```python
from build123d import *

# Parameters (mm, degrees)
SKETCH1_R           = 2
BOSS_EXTRUDE1_DEPTH = 3
SKETCH2_R           = 0.75
CUT_EXTRUDE1_DEPTH  = 17.126356976


with BuildPart() as part:
    # Sketch1 → Boss-Extrude1 (new body)
    with BuildSketch(Plane(origin=(0, 0, 0), x_dir=(0, 0, -1), z_dir=(1, 0, 0))):
        with BuildLine():
            Line((-4, 10), (-4, 0))
            ThreePointArc((-4, 0), (-0.694592711, -3.939231012), (3.758770483, -1.368080573))
            Line((3.758770483, -1.368080573), (7.178971916, 8.028845635))
            ThreePointArc((7.178971916, 8.028845635), (7.045432581, 11.087399255), (4.788282007, 13.155696691))
            ThreePointArc((4.788282007, 13.155696691), (2.431074487, 13.787308542), (0, 14))
            ThreePointArc((0, 14), (-2.828427125, 12.828427125), (-4, 10))
        make_face()
        Circle(SKETCH1_R, mode=Mode.SUBTRACT)
        with Locations((0, 10)):
            Circle(SKETCH1_R, mode=Mode.SUBTRACT)
    extrude(amount=BOSS_EXTRUDE1_DEPTH)

    # Sketch2 → Cut-Extrude1 (cut, through all)
    with BuildSketch(Plane(origin=(3, 0, 0), x_dir=(0, 0, -1), z_dir=(1, 0, 0))):
        with Locations((5, 8)):
            Circle(SKETCH2_R)
    extrude(amount=-CUT_EXTRUDE1_DEPTH, mode=Mode.SUBTRACT)


solid = part.part
```
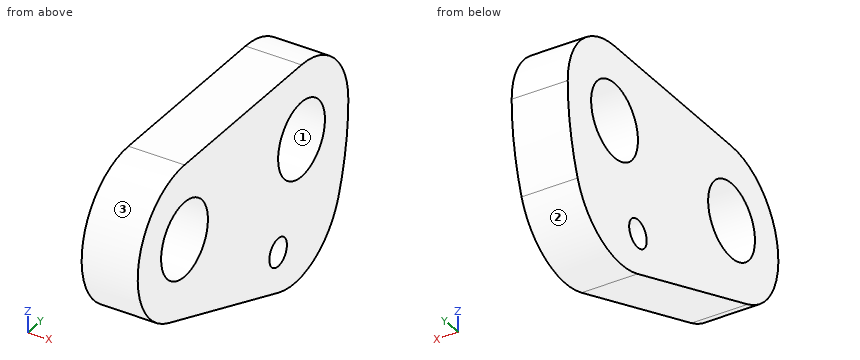
Geometry check sheet. Reference: the model listing, model coordinates, mm. Face numbers are marked on the shaded views. Coordinates: 2 decimals unless noted, no trailing zeros. Order: outer loops, then holes, each group sorted by start corner. A loop starts at its lowest first (then second) coordinate and runs counter-clockwise, first axis right, second up.
Q1. Sectioned sample at B-B on z = -1.5. Record the cut outline in (x, y).
Reply:
outline: (0, -3.71) - (3, -3.71) - (3, -1.32) - (0, -1.32) - close; (0, 1.32) - (3, 1.32) - (3, 8.68) - (0, 8.68) - close; (0, 11.32) - (3, 11.32) - (3, 13.92) - (0, 13.92) - close
Q2. Sectioned sample at D-D on z = -5. Record the cut outline in (x, y).
Reply:
outline: (0, 2.04) - (3, 2.04) - (3, 7.25) - (0, 7.25) - close; (0, 8.75) - (3, 8.75) - (3, 13.07) - (0, 13.07) - close
Q3. Sectioned sample at C-C on y = 0.5. Record the cut outline in (x, z), and give its area (3 significant figures).
Reply:
outline: (0, -4.44) - (3, -4.44) - (3, -1.94) - (0, -1.94) - close; (0, 1.94) - (3, 1.94) - (3, 4) - (0, 4) - close
area: 13.7 mm2
Q4. Depth check by flat-ended pin: pin 1 Ø1 at (x, y) = (1, 0.5) entering from -Z; pin 2 Ø1.5 at (x, z) = (1, -4.5) entering from +Y; pin 3 Ø0.9 at (y, z) = (8, -5) entering from -X. Enter the tip coordinate at first touch or a pass-through.
Reply:
pin 1: stops at z = -4.62
pin 2: stops at y = 13.49
pin 3: passes through
Q5. Draft check along Z on the marked faces 1, 2 and 3. Enter one of: released by +Z, released by -Z, zero draft, split by the parting line, or undercut.
Reply:
face 1: undercut
face 2: released by -Z
face 3: split by the parting line
Q6. Sectioned sample at A-A on x = 0.65. Record the cut outline in (y, z), and give its area (3 significant figures).
Reply:
outline: (-1.37, -3.76) - (8.03, -7.18) arc R4 ccw to (13.16, -4.79) arc R14 ccw to (14, 0) arc R4 ccw to (10, 4) - (0, 4) arc R4 ccw to start; hole circle Ø4 at (0, 0); hole circle Ø1.5 at (8, -5); hole circle Ø4 at (10, 0)
area: 135 mm2
Q7. Thickness scan on probe 1 along Y at (x, z) = (2.5, -0.5); probe 2 along Y at (x, z) = (1.8, 1.25); probe 3 along Z at (x, y) = (2.85, 1). Record the ranges inside material, lowest first.
Reply:
probe 1: y = -3.97 to -1.94, 1.94 to 8.06, 11.94 to 13.99
probe 2: y = -3.8 to -1.56, 1.56 to 8.44, 11.56 to 13.8
probe 3: z = -4.62 to -1.73, 1.73 to 4
